Read the model definition and answer for the solid it produces. Units are mm, in the model's axes. A direction names the side the tool comes from. Coordinates: 2 decimals unless noted, no trailing zeros. Write each loop counter-clockwise with the first axis right and the second up, starting at its lowest first coordinate (ties: lowest second). Pieces come first, ordered by that corner, then holes. Notation, with made-up numbers: (-17, -28.75) -> (5, -28.75) arc R7 cw to (5, -22.75) -> close; hole circle Ø4 at (79.25, 64). An arc over 180 degrees is marked (long way). Use CSV: the item, a comma, the result in double quotes.
from build123d import *

# Parameters (mm, degrees)
CYLINDER025_R             = 41.25
CYLINDER025_DEPTH         = 1.5
BOX002_W                  = 16.9
BOX002_H                  = 4
BOX002_DEPTH              = 1.5
BOX003_W                  = 16.9
BOX003_H                  = 4
BOX003_DEPTH              = 1.5
FUSION008_PLACEMENT_ANGLE = 22.5
CYLINDER018_R             = 35
CYLINDER018_DEPTH         = 10.6
CYLINDER019_R             = 31
CYLINDER019_DEPTH         = 17
CYLINDER023_R             = 4.2
CYLINDER023_DEPTH         = 17
ARRAY004_COUNT            = 8
CYLINDER022_R             = 38.6
CYLINDER022_DEPTH         = 0.22
CYLINDER021_R             = 41.25
CYLINDER021_DEPTH         = 1.2
CYLINDER020_R             = 57.15
CYLINDER020_DEPTH         = 17


with BuildPart() as cylinder025:
    # Cylinder025 → Cylinder025 (new body)
    with BuildSketch(Plane.XY):
        Circle(CYLINDER025_R)
    extrude(amount=CYLINDER025_DEPTH)


with BuildPart() as cube002:
    # Box002 → Box002 (new body)
    with BuildSketch(Plane(origin=(40.75, -2, 0), x_dir=(1, 0, 0), z_dir=(0, 0, 1))):
        with Locations((8.45, 2)):
            Rectangle(BOX002_W, BOX002_H)
    extrude(amount=BOX002_DEPTH)


with BuildPart() as obj1:
    # Box003 → Box003 (new body)
    with BuildSketch(Plane(origin=(-57.65, -2, 0), x_dir=(1, 0, 0), z_dir=(0, 0, 1))):
        with Locations((8.45, 2)):
            Rectangle(BOX003_W, BOX003_H)
    extrude(amount=BOX003_DEPTH)

    # Fusion008: union Cube002
    add(cube002.part)


with BuildPart() as obj1_1:
    # Fusion008 placement: moved
    add(obj1.part.rotate(Axis((0, 0, 0), (0, 0, 1)), FUSION008_PLACEMENT_ANGLE))

    # Cut021: cut Cylinder025
    add(cylinder025.part, mode=Mode.SUBTRACT)


with BuildPart() as cylinder018:
    # Cylinder018 → Cylinder018 (new body)
    with BuildSketch(Plane.XY.offset(6.4)):
        Circle(CYLINDER018_R)
    extrude(amount=CYLINDER018_DEPTH)


with BuildPart() as fusion006:
    # Cylinder019 → Cylinder019 (new body)
    with BuildSketch(Plane.XY):
        Circle(CYLINDER019_R)
    extrude(amount=CYLINDER019_DEPTH)

    # Fusion006: union Cylinder018
    add(cylinder018.part)


with BuildPart() as boltholearray004:
    # Cylinder023 → Cylinder023 (new body)
    with BuildSketch(Plane(origin=(46.1, 0, 0), x_dir=(1, 0, 0), z_dir=(0, 0, 1))):
        Circle(CYLINDER023_R)
    extrude(amount=CYLINDER023_DEPTH)

    # Array004: BoltHoleArray004 ×8 about axis
    array004_axis = Axis((0, 0, 0), (0, 0, 1))


with BuildPart() as boltholearray004_1:
    add(boltholearray004.part)
    for i in range(1, ARRAY004_COUNT):
        add(boltholearray004.part.rotate(array004_axis, i * 360 / ARRAY004_COUNT))


with BuildPart() as cylinder022:
    # Cylinder022 → Cylinder022 (new body)
    with BuildSketch(Plane.XY):
        Circle(CYLINDER022_R)
    extrude(amount=CYLINDER022_DEPTH)


with BuildPart() as knifeedge004:
    # Cone004 → Cone004 (revolve)
    with BuildSketch(Plane.XZ):
        Polygon((0, 0), (38.6, 0), (41.25, 0.22), (0, 0.22), align=None)
    revolve(axis=Axis((0, 0, 0), (0, 0, 1)))

    # Cut016: cut Cylinder022
    add(cylinder022.part, mode=Mode.SUBTRACT)


with BuildPart() as knifeedge004_1:
    # Cut016 placement: moved
    add(knifeedge004.part.moved(Location((0, 0, 0.98))))


with BuildPart() as sealrecess004:
    # Cylinder021 → Cylinder021 (new body)
    with BuildSketch(Plane.XY):
        Circle(CYLINDER021_R)
    extrude(amount=CYLINDER021_DEPTH)


with BuildPart() as obj2:
    # Cylinder020 → Cylinder020 (new body)
    with BuildSketch(Plane.XY):
        Circle(CYLINDER020_R)
    extrude(amount=CYLINDER020_DEPTH)

    # Cut015: cut SealRecess004
    add(sealrecess004.part, mode=Mode.SUBTRACT)

    # Fusion005: union KnifeEdge004
    add(knifeedge004_1.part)

    # Cut017: cut BoltHoleArray004
    add(boltholearray004_1.part, mode=Mode.SUBTRACT)

    # Cut018: cut Fusion006
    add(fusion006.part, mode=Mode.SUBTRACT)

    # Cut024: cut obj1
    add(obj1_1.part, mode=Mode.SUBTRACT)


solid = obj2.part
1. A cutting plane is placed at D-D (x = -46.1). Give the vertices of the cut face in (y, z), and give its area (3 significant figures).
Solutions:
outline,"(-33.78, 0) -> (-21.26, 0) -> (-21.26, 1.5) -> (-16.93, 1.5) -> (-16.93, 0) -> (-4.2, 0) -> (-4.2, 17) -> (-33.78, 17) -> close; (4.2, 0) -> (33.78, 0) -> (33.78, 17) -> (4.2, 17) -> close"
area,"999 mm^2"
2. Each of these flat-tipped pins is pushed along its axis until it touches: pin 1 Ø6 at (y, z) = (27, 11.5) entering from -X; pin 2 Ø5 at (x, z) = (-20, 2) entering from +Y; pin 3 Ø1.5 at (y, z) = (17.5, 15) entering from +X. Where does it stop, or does it pass through?
Solutions:
pin 1,"stops at x = -51.87"
pin 2,"stops at y = 54.4"
pin 3,"stops at x = 54.64"
3. A cutting plane is placed at C-C (y = 46.1). Give the vertices of the cut face in (x, z), and give its area (3 significant figures).
Solutions:
outline,"(-33.78, 0) -> (-4.2, 0) -> (-4.2, 17) -> (-33.78, 17) -> close; (4.2, 0) -> (33.78, 0) -> (33.78, 17) -> (4.2, 17) -> close"
area,"1,010 mm^2"
4. For a pull along X with two mould halves and no side action, classify faces 1 (the cylindrical face through (-57.095, 2.513, 8.381)), 2 (the cylindrical face through (0.185, -41.904, 8.381)), 3 (the flat face through (-26, -25, 17)), 4 (the cylindrical face through (-0.185, 41.904, 8.381)) as pulls with the +X half, pulls with the -X half, needs draft (parallel to the pull), parting line crosses it, or undercut.
Solutions:
face 1,"parting line crosses it"
face 2,"undercut"
face 3,"needs draft"
face 4,"undercut"
5. A tool of negligible diameter and unlimited length cuts with its end or side. For faces 5 (the cylindrical face through (-4.036, 30.736, 3.764)), 6 (the flat face through (-20.9, -23.2, 6.4)), 7 (the flat face through (-44.75, -20.7, 0.74)), from which of +Z, -Z, +X, -X, +Y, -Y can it reach the whole face along a straight path? Write none if from no direction.
Solutions:
face 5,"+Z, -Z"
face 6,"+Z"
face 7,"-Z"
6. Find the intervals of material crossed by line 1 along X through (y, z) = (1.5, 11.75); line 2 along X through (y, z) = (-26, 11.75); line 3 along X through (y, z) = (-21.5, 4.25), in increasing order.
Solutions:
line 1,"x = -57.13 to -50.02, -42.18 to -34.97, 34.97 to 42.18, 50.02 to 57.13"
line 2,"x = -50.89 to -23.43, 23.43 to 50.89"
line 3,"x = -52.95 to -22.33, 22.33 to 52.95"
7. A cutting plane is placed at A-A (y = 0). Give the vertices of the cut face in (x, z), and give its area (3 significant figures).
Solutions:
outline,"(-57.15, 0) -> (-50.3, 0) -> (-50.3, 17) -> (-57.15, 17) -> close; (-41.9, 0) -> (-41.25, 0) -> (-41.25, 1.2) -> (-38.6, 0.98) -> (-38.6, 1.2) -> (-31, 1.2) -> (-31, 6.4) -> (-35, 6.4) -> (-35, 17) -> (-41.9, 17) -> close; (31, 1.2) -> (38.6, 1.2) -> (38.6, 0.98) -> (41.25, 1.2) -> (41.25, 0) -> (41.9, 0) -> (41.9, 17) -> (35, 17) -> (35, 6.4) -> (31, 6.4) -> close; (50.3, 0) -> (57.15, 0) -> (57.15, 17) -> (50.3, 17) -> close"
area,"495 mm^2"
